Design review of the part built by this model. Coordinates are the model's own, in mm. Coordinates: 2 decimals unless noted, no trailing zeros. Write each loop counter-clockwise with the first axis right and the second up, starting at its lowest first coordinate (ties: lowest second). Pieces come first, ordered by that corner, then holes. Notation, with made-up numbers: (83, 4) - (90, 4) arc R28 ccw to (90, 38) - close; hole circle Ø8 at (81, 10.25). An arc over 180 degrees is marked (long way). Answer as a JSON object with one key per item and string values.
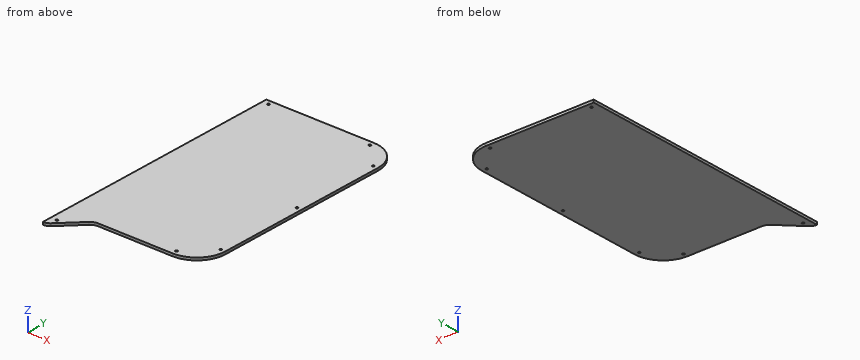
```python
from build123d import *

# Parameters (mm, degrees)
SKETCH1_R           = 1.75
BOSS_EXTRUDE1_DEPTH = 4


with BuildPart() as part:
    # Sketch1 → Boss-Extrude1 (new body)
    with BuildSketch(Plane.XY):
        with BuildLine():
            Line((2024.321699886, -20.389970185), (2025.564078039, -20.389970185))
            ThreePointArc((2025.564078039, -20.389970185), (2030.155451072, -19.476867572), (2034.048091653, -16.876519131))
            Line((2034.048091653, -16.876519131), (2066.152417854, 15.218215997))
            ThreePointArc((2066.152417854, 15.218215997), (2071.01821858, 18.468651549), (2076.757434871, 19.610029815))
            Line((2076.757434871, 19.610029815), (2193.821699886, 19.610029815))
            ThreePointArc((2193.821699886, 19.610029815), (2225.64150504, 32.790224661), (2238.821699886, 64.610029815))
            Line((2238.821699886, 64.610029815), (2238.821699886, 344.610029815))
            ThreePointArc((2238.821699886, 344.610029815), (2225.64150504, 376.429834968), (2193.821699886, 389.610029815))
            Line((2193.821699886, 389.610029815), (2024.321699886, 389.610029815))
            Line((2024.321699886, 389.610029815), (2024.321699886, -20.389970185))
        make_face()
        with Locations((2034.048091653, -6.27150164)):
            Circle(SKETCH1_R, mode=Mode.SUBTRACT)
        with Locations((2193.821699886, 27.110029815)):
            Circle(SKETCH1_R, mode=Mode.SUBTRACT)
        with Locations((2231.321699886, 64.610029815)):
            Circle(SKETCH1_R, mode=Mode.SUBTRACT)
        with Locations((2231.321699886, 204.610029815)):
            Circle(SKETCH1_R, mode=Mode.SUBTRACT)
        with Locations((2231.321699886, 344.610029815)):
            Circle(SKETCH1_R, mode=Mode.SUBTRACT)
        with Locations((2193.821699886, 382.110029815)):
            Circle(SKETCH1_R, mode=Mode.SUBTRACT)
        with Locations((2034.048091653, 382.110029815)):
            Circle(SKETCH1_R, mode=Mode.SUBTRACT)
    extrude(amount=BOSS_EXTRUDE1_DEPTH)


solid = part.part
```
(1) Take a section at C-C, the plane y = 44. Write out the cut boundary in (x, z).
Solved:
{"outline": "(2024.32, 0) - (2233.82, 0) - (2233.82, 4) - (2024.32, 4) - close"}
(2) To check wall thickness, follow line 1 (Y direction, x = 2195, z = 3.7); line 2 (X direction, y = 66, z = 2.05); line 3 (Y direction, x = 2148, z = 1.1). State the ranges of each line that lie inside material, in increasing order. Write a range as from..to.
Solved:
{"line 1": "y = 19.63..25.82, 28.4..380.82, 383.4..389.59", "line 2": "x = 2024.32..2230.26, 2232.38..2238.82", "line 3": "y = 19.61..389.61"}
(3) For pin 1 (1 mm diameter, centred on x = 2200.5, z = 3, fed in from +Y); pin 2 (2 mm diameter, centred on x = 2138, z = 3, fed in from -Y), all flat-tipped, find the tip position at first contact; note any pin that passes through.
Solved:
{"pin 1": "stops at y = 389.18", "pin 2": "stops at y = 19.61"}
(4) Take a section at A-A, the plane z = 1.35. Write out the cut boundary in (x, y), and give its area (3 significant figures).
Solved:
{"outline": "(2024.32, -20.39) - (2025.56, -20.39) arc R12 ccw to (2034.05, -16.88) - (2066.15, 15.22) arc R15 cw to (2076.76, 19.61) - (2193.82, 19.61) arc R45 ccw to (2238.82, 64.61) - (2238.82, 344.61) arc R45 ccw to (2193.82, 389.61) - (2024.32, 389.61) - close; hole circle Ø3.5 at (2034.05, -6.27); hole circle Ø3.5 at (2034.05, 382.11); hole circle Ø3.5 at (2193.82, 27.11); hole circle Ø3.5 at (2193.82, 382.11); hole circle Ø3.5 at (2231.32, 64.61); hole circle Ø3.5 at (2231.32, 204.61); hole circle Ø3.5 at (2231.32, 344.61)", "area": "79,500 mm^2"}
(5) Take a section at B-B, the plane x = 2146. Write out the cut boundary in (y, z), and give its area (3 significant figures).
Solved:
{"outline": "(19.61, 0) - (389.61, 0) - (389.61, 4) - (19.61, 4) - close", "area": "1,480 mm^2"}
